Geometry check sheet. Reference: the model listing, model coordinates, mm. A direction names the side the tool comes from. Give positions to 0.01 mm unless a question says otherwise; leave off trailing zeros. Write each loop counter-clockwise with the first axis right and the second up, starting at its lowest first coordinate (ties: lowest second). Pieces come first, ordered by that corner, then holes. Notation, with made-up numbers: M -39.75,15.25 L 8.25,15.25 A18 ccw 8.25,44.25 Z; hole C 55.25,-31.5 d5. An arc over 180 degrees is marked long. Use one line per item in the form item = value. Start each with the question number.
```python
from build123d import *

# Parameters (mm, degrees)
ESQUISSE1_W             = 3
ESQUISSE1_H             = 2.8
ENL_V_MAT_EXTRU_1_DEPTH = 21
ESQUISSE2_R             = 8
ENL_V_MAT_EXTRU_2_DEPTH = 1


with BuildPart() as part:
    # Sketch1 → Revolve2 (revolve)
    with BuildSketch(Plane.XY):
        with BuildLine():
            Line((5, -15), (8, -15))
            Line((8, -15), (8, -5))
            Line((8, -5), (11.5, -5))
            Line((11.5, -5), (11.5, -2.598076211))
            ThreePointArc((11.5, -2.598076211), (11, 0), (11.5, 2.598076211))
            Line((11.5, 2.598076211), (11.5, 5))
            Line((11.5, 5), (5, 5))
            Line((5, 5), (5, -15))
        make_face()
    revolve(axis=Axis((0, -15, 0), (0, 1, 0)))

    # Esquisse1 → Enlèv. mat.-Extru.1 (cut, through all)
    with BuildSketch(Plane(origin=(0, 5, 0), x_dir=(1, 0, 0), z_dir=(0, 1, 0))):
        with Locations((0, 5)):
            Rectangle(ESQUISSE1_W, ESQUISSE1_H)
    extrude(amount=-ENL_V_MAT_EXTRU_1_DEPTH, mode=Mode.SUBTRACT)

    # Esquisse2 → Enlèv. mat.-Extru.2 (cut)
    with BuildSketch(Plane.XZ.offset(15)):
        Circle(ESQUISSE2_R)
    extrude(amount=-ENL_V_MAT_EXTRU_2_DEPTH, mode=Mode.SUBTRACT)


solid = part.part
```
(1) Sectioned sample at B-B, the plane y = -8.5. Record the boundary of the cut face in (x, z), plus the area to 3 significant figures.
(2) Draft check along X on faces 4 (the flat face through (5.2, -14, 0.1)), 5 (the cylindrical face through (0, -5, 5)), 6 (the cylindrical face through (-1.73, -9.44, 7.81)), 7 (the flat face through (1.5, -4, -6)). Enter one of: released by +X, released by -X, zero draft, split by the parting line, or undercut.
(3) Sectioned sample at C-C, the plane z = 0. Record the boundary of the cut face in (x, y).
(4) Depth check by flat-ended pin: pin 1 (1.3 mm diameter, centred on y = -6, z = -5.5, fed in from +X); pin 2 (2 mm diameter, centred on x = -6.5, y = -3.5, fed in from -Z); pin 3 (4 mm diameter, centred on y = -8.5, z = -6.5, fed in from +X). Enter the tip coordinate at first touch or a pass-through.
(5) Sectioned sample at A-A, the plane x = 0. Record the boundary of the cut face in (y, z), plus the area to 3 significant figures.
(6) Thickness scan on probe 1 along X at (y, z) = (-3.5, 0); probe 2 along Z at (x, y) = (-6.25, -8.25); probe 3 along X at (y, z) = (-5.25, 0). Record the ranges inside material, lowest first. Write a range as [from, to].
(7) Sectioned sample at D-D, the plane y = 3. Record the boundary of the cut face in (x, z).
(8) Tool access check on faces 1 (the flat face through (2, 5, 5)), 2 (the flat face through (-1.5, -4, -6)), 3 (the flat face through (8, -5, 2)). Record the directions out of +Z, -Z, +X, -X, +Y, -Y that give a thin tool (end or side, any length) a straight path to the whole face; none if there is none.
Numbers:
q1.outline = C 0,0 d16; hole M -1.5,-6.4 L 1.5,-6.4 L 1.5,-4.77 A5 ccw long -1.5,-4.77 Z
q1.area = 118 mm2
q2.face_4 = zero draft
q2.face_5 = undercut
q2.face_6 = split by the parting line
q2.face_7 = undercut
q3.outline = M -11.5,-5 L -8,-5 L -8,-14 L -5,-14 L -5,5 L -11.5,5 L -11.5,2.6 A7 cw -11.5,-2.6 Z; M 5,-14 L 8,-14 L 8,-5 L 11.5,-5 L 11.5,-2.6 A7 cw 11.5,2.6 L 11.5,5 L 5,5 Z
q4.pin_1 = 6.36
q4.pin_2 = -10.1
q4.pin_3 = 6.61
q5.outline = M -14,-8 L -5,-8 L -5,-11.5 L -2.6,-11.5 A7 cw 2.6,-11.5 L 5,-11.5 L 5,-6.4 L -14,-6.4 Z; M -14,5 L 5,5 L 5,11.5 L 2.6,11.5 A7 cw -2.6,11.5 L -5,11.5 L -5,8 L -14,8 Z
q5.area = 154 mm2
q6.probe_1 = [-11.5, -5], [5, 11.5]
q6.probe_2 = [-4.99, 4.99]
q6.probe_3 = [-8, -5], [5, 8]
q7.outline = C 0,0 d23; hole M -1.5,-6.4 L 1.5,-6.4 L 1.5,-4.77 A5 ccw long -1.5,-4.77 Z
q8.face_1 = +Z, -Z, +X, -X, +Y
q8.face_2 = +Y, -Y
q8.face_3 = -Y
